Verification items for the finished model (mm, model axes). A direction names the side the tool comes from. Coordinates: 2 decimals unless noted, no trailing zeros. Order: outer loops, then holes, each group sorted by start corner. A loop starts at its lowest first (then second) coordinate and runs counter-clockwise, first axis right, second up. Notation, with made-up numbers: M -14,72 L 6,72 A26 ccw 6,98 Z; hole C -38.5,82 d7. An arc over 180 degrees is marked long. Write item = value, one per line.
```python
from build123d import *

# Parameters (mm, degrees)
SKETCH_1_W          = 28
SKETCH_1_H          = 23
EXTRUDE_1_DEPTH     = 1.5
SKETCH_2_W          = 28
SKETCH_2_H          = 23
SKETCH_2_W_2        = 25
SKETCH_2_H_2        = 20
EXTRUDE_2_DEPTH     = 5
SKETCH_4_W          = 10
SKETCH_4_H          = 2
CUT_EXTRUDE_1_DEPTH = 2
SKETCH_5_W          = 5
SKETCH_5_H          = 33
EXTRUDE_3_DEPTH     = 2.5
SKETCH_6_W          = 5
SKETCH_6_H          = 20
CUT_EXTRUDE_2_DEPTH = 1
SKETCH_7_R          = 1
CUT_EXTRUDE_3_DEPTH = 40.799497484
FILLET_1_R          = 2


with BuildPart() as part:
    # 草图1 → 凸台-拉伸1 (new body)
    with BuildSketch(Plane(origin=(0, 0, 0), x_dir=(1, 0, 0), z_dir=(0, 1, 0))):
        with Locations((14, -11.5)):
            Rectangle(SKETCH_1_W, SKETCH_1_H)
    extrude(amount=EXTRUDE_1_DEPTH)

    # 草图2 → 凸台-拉伸2 (add)
    with BuildSketch(Plane(origin=(0, 1.5, 0), x_dir=(1, 0, 0), z_dir=(0, 1, 0))):
        with Locations((14, -11.5)):
            Rectangle(SKETCH_2_W, SKETCH_2_H)
        with Locations((14, -11.5)):
            Rectangle(SKETCH_2_W_2, SKETCH_2_H_2, mode=Mode.SUBTRACT)
    extrude(amount=EXTRUDE_2_DEPTH)

    # 草图4 → 切除-拉伸1 (cut)
    with BuildSketch(Plane(origin=(28, 0, 0), x_dir=(0, 0, -1), z_dir=(1, 0, 0))):
        with Locations((-11.5, 5.5)):
            Rectangle(SKETCH_4_W, SKETCH_4_H)
    extrude(amount=-CUT_EXTRUDE_1_DEPTH, mode=Mode.SUBTRACT)

    # 草图5 → 凸台-拉伸3 (add)
    with BuildSketch(Plane.XZ):
        with Locations((14, 11.5)):
            Rectangle(SKETCH_5_W, SKETCH_5_H)
    extrude(amount=-EXTRUDE_3_DEPTH)

    # 草图6 → 切除-拉伸2 (cut)
    with BuildSketch(Plane(origin=(0, 2.5, 0), x_dir=(1, 0, 0), z_dir=(0, 1, 0))):
        with Locations((14, -11.5)):
            Rectangle(SKETCH_6_W, SKETCH_6_H)
    extrude(amount=-CUT_EXTRUDE_2_DEPTH, mode=Mode.SUBTRACT)

    # 草图7 → 切除-拉伸3 (cut, through all)
    with BuildSketch(Plane(origin=(0, 2.5, 0), x_dir=(1, 0, 0), z_dir=(0, 1, 0))):
        with Locations(Location((14, 2.5, 0), (0, 0, 270))):
            Circle(SKETCH_7_R)
        with Locations(Location((14, -25.5, 0), (0, 0, 270))):
            Circle(SKETCH_7_R)
    extrude(amount=-CUT_EXTRUDE_3_DEPTH, mode=Mode.SUBTRACT)

    # 圆角1
    fillet_1_edges = [part.edges().sort_by_distance(p)[0] for p in [
        (11.5, 1.25, -5),
        (16.5, 1.25, 28),
        (11.5, 1.25, 28),
        (16.5, 1.25, -5),
    ]]
    fillet(fillet_1_edges, radius=FILLET_1_R)


solid = part.part
```
Item 1: Sectioned sample at D-D, the plane y = 1. Enter the section's corners in (x, z).
Report:
outline = M 0,0 L 11.5,0 L 11.5,-3 A2 ccw 13.5,-5 L 14.5,-5 A2 ccw 16.5,-3 L 16.5,0 L 28,0 L 28,23 L 16.5,23 L 16.5,26 A2 ccw 14.5,28 L 13.5,28 A2 ccw 11.5,26 L 11.5,23 L 0,23 Z; hole C 14,-2.5 d2; hole C 14,25.5 d2
Item 2: Tool access check on faces 1 (the flat face through (0, 3, 12)), 2 (the flat face through (14, 2.5, 24)), 3 (the flat face through (14, 1.5, 11)), 4 (the flat face through (27, 5, 6.5)), 5 (the flat face through (11.5, 1, 24)). Record the directions out of +Z, -Z, +X, -X, +Y, -Y that give a thin tool (end or side, any length) a straight path to the whole face; none if there is none.
Report:
face_1 = +Z, -Z, -X, +Y, -Y
face_2 = +Z, +X, -X, +Y
face_3 = +Y
face_4 = +X, +Y
face_5 = +Z, -X, +Y, -Y
Item 3: Sectioned sample at B-B, the plane y = 3.5. Enter the section's corners in (x, z).
Report:
outline = M 0,0 L 28,0 L 28,23 L 0,23 Z; hole M 1.5,1.5 L 26.5,1.5 L 26.5,21.5 L 1.5,21.5 Z
Item 4: Scan lines: L1, parallel to X at y = 4, z = 2.5; L2, parallel to Z at x = 4.5, y = 3.5; L3, parallel to X at y = 1.45, z = 25.5. Record each from-to range of solid material in increasing order. Write a range as from..to.
Report:
L1 = 0..1.5, 26.5..28
L2 = 0..1.5, 21.5..23
L3 = 11.5..13, 15..16.5
Item 5: Sectioned sample at A-A, the plane x = 14. Enter the section's corners in (y, z), then the cut area to 3 significant figures.
Report:
outline = M 0,-5 L 2.5,-5 L 2.5,-3.5 L 0,-3.5 Z; M 0,-1.5 L 2.5,-1.5 L 2.5,0 L 6.5,0 L 6.5,1.5 L 1.5,1.5 L 1.5,21.5 L 6.5,21.5 L 6.5,23 L 2.5,23 L 2.5,24.5 L 0,24.5 Z; M 0,26.5 L 2.5,26.5 L 2.5,28 L 0,28 Z
area = 64.5 mm^2
Item 6: Gauge pin test, flat ends, axial feed: pin 1 (3 mm diameter, centred on x = 14, z = -2.5, fed in from +Y); pin 2 (1.2 mm diameter, centred on y = 0.5, z = 24.5, fed in from +X); pin 3 (12 mm diameter, centred on x = 10.5, z = 11.5, fed in from +Y). Record the tip position at first contact, or that the pin passes through.
Report:
pin_1 = 2.5
pin_2 = 16.5
pin_3 = 1.5
Item 7: Sectioned sample at C-C, the plane z = -2.5. Enter the section's corners in (x, y), then the cut area to 3 significant figures.
Report:
outline = M 11.5,0 L 13,0 L 13,2.5 L 11.5,2.5 Z; M 15,0 L 16.5,0 L 16.5,2.5 L 15,2.5 Z
area = 7.50 mm^2
Item 8: Release check for a two-part mould opening along X. For faces 6 (the cylindrical face through (15.9, 1.27, 27.43)), 7 (the flat face through (14, 4, 1.5)), 8 (the flat face through (11.5, 1, -2)), 9 (the flat face through (14, 4, 21.5)) record: pulls with the +X half, pulls with the -X half, needs draft (parallel to the pull), parting line crosses it, or undercut.
Report:
face_6 = pulls with the +X half
face_7 = undercut
face_8 = pulls with the -X half
face_9 = undercut
